```python
from build123d import *

# Parameters (mm, degrees)
BOSS_EXTRUDE1_DEPTH   = 10
SKETCH1_W             = 30
SKETCH1_H             = 3
BOSS_EXTRUDE1_2_DEPTH = 10
BOSS_EXTRUDE2_DEPTH   = 4.8
BOSS_EXTRUDE3_START   = 5.2
BOSS_EXTRUDE3_DEPTH   = 4.8
FILLET1_R             = 0.5
CUT_EXTRUDE1_REACH    = 55.298


with BuildPart() as part:
    # Sketch1 → Boss-Extrude1 (new, symmetric)
    with BuildSketch(Plane(origin=(0, 0, 0), x_dir=(0, 0, -1), z_dir=(1, 0, 0))):
        with BuildLine():
            Line((0, 13), (0, 11.2))
            Line((0, 11.2), (4.930378913, 10.768647738))
            Line((4.930378913, 10.768647738), (24, 13.896674439))
            Line((24, 13.896674439), (42, 13.896674439))
            ThreePointArc((42, 13.896674439), (43.5, 15.396674439), (42, 16.896674439))
            Line((42, 16.896674439), (23.755585281, 16.896674439))
            Line((23.755585281, 16.896674439), (0, 13))
        make_face()
    extrude(amount=BOSS_EXTRUDE1_DEPTH, both=True)



with BuildPart() as body_2:
    # Sketch1 → Boss-Extrude1 2 (new, symmetric)
    with BuildSketch(Plane(origin=(0, 0, 0), x_dir=(0, 0, -1), z_dir=(1, 0, 0))):
        with Locations((33, -2.5)):
            Rectangle(SKETCH1_W, SKETCH1_H)
    extrude(amount=BOSS_EXTRUDE1_2_DEPTH, both=True)


with BuildPart() as part_1:
    add(part.part)

    add(body_2.part)  # Boss-Extrude2 merges body 2
    # Sketch2 → Boss-Extrude2 (add, symmetric)
    with BuildSketch(Plane(origin=(0, 0, 0), x_dir=(0, 0, -1), z_dir=(1, 0, 0))):
        Polygon((30.537640136, 13.896674439), (45.434314575, -1), (46.565685425, -1), (31.669010986, 13.896674439), align=None)
    extrude(amount=BOSS_EXTRUDE2_DEPTH, both=True)

    # Sketch3 → Boss-Extrude3 (add)
    with BuildSketch(Plane(origin=(0, 0, 0), x_dir=(0, 0, -1), z_dir=(1, 0, 0)).offset(BOSS_EXTRUDE3_START)):
        Polygon((19.434314575, -1), (20.565685425, -1), (35.462359864, 13.896674439), (34.330989014, 13.896674439), align=None)
    boss_extrude3 = extrude(amount=BOSS_EXTRUDE3_DEPTH)

    # Mirror1: Boss-Extrude3 across plane
    add(boss_extrude3.mirror(Plane(origin=(0, 0, 0), x_dir=(0, 0, 1), z_dir=(1, 0, 0))))

    # Fillet1
    fillet1_edges = [part_1.edges().sort_by_distance(p)[0] for p in [
        (0, 13.896674439, -31.669010986),
        (0, 13.896674439, -30.537640136),
        (0, -1, -45.434314575),
        (0, -1, -46.565685425),
        (7.6, -1, -20.565685425),
        (7.6, 13.896674439, -35.462359864),
        (7.6, 13.896674439, -34.330989014),
        (7.6, -1, -19.434314575),
        (-7.6, -1, -20.565685425),
        (-7.6, -1, -19.434314575),
    ]]
    fillet(fillet1_edges, radius=FILLET1_R)

    # Sketch4 → Cut-Extrude1 (cut, up to next)
    with BuildSketch(Plane(origin=(0, 16.896674439, 0), x_dir=(1, 0, 0), z_dir=(0, 1, 0)), mode=Mode.PRIVATE) as cut_extrude1_sk1:
        Polygon((-3, 0), (-10, 26.585294569), (-10, 0), align=None)
    cut_extrude1_tool1 = extrude(cut_extrude1_sk1.sketch, amount=-CUT_EXTRUDE1_REACH, mode=Mode.PRIVATE) & part_1.part
    # Sketch4 → Cut-Extrude1 (cut, up to next)
    with BuildSketch(Plane(origin=(0, 16.896674439, 0), x_dir=(1, 0, 0), z_dir=(0, 1, 0)), mode=Mode.PRIVATE) as cut_extrude1_sk2:
        Polygon((3, 0), (10, 0), (10, 26.585294569), align=None)
    cut_extrude1_tool2 = extrude(cut_extrude1_sk2.sketch, amount=-CUT_EXTRUDE1_REACH, mode=Mode.PRIVATE) & part_1.part
    add(cut_extrude1_tool1.solids().sort_by_distance((-7.666667, 16.896674, -8.861765))[0], mode=Mode.SUBTRACT)
    add(cut_extrude1_tool2.solids().sort_by_distance((7.666667, 16.896674, -8.861765))[0], mode=Mode.SUBTRACT)


solid = part_1.part
```
Could you check a few things on this model? Use its own coordinates, in mm. A direction names the side the tool comes from. Coordinates: 2 decimals unless noted, no trailing zeros. Write each loop counter-clockwise with the first axis right and the second up, starting at its lowest first coordinate (ties: lowest second). Pieces come first, ordered by that corner, then holes. Notation, with made-up numbers: (57, -37.5) -> (116, -37.5) arc R32 ccw to (116, -11.5) -> close; hole circle Ø7 at (44.5, -20.75). An arc over 180 degrees is marked (long way). One line per question, with ' | ' between items. Start each with the question number.
1. Thinking about a two-plate mould opening in X: for faces 4 (the face through (-10, 7, -28)), 5 (the face through (5.2, 6, -27)), 6 (the face through (0.067, -0.699, -44.686)), 7 (the face through (-5.2, 6, -27)), which applies, pulls with the +X half, pulls with the -X half, needs draft (parallel to the pull), parting line crosses it, or undercut?
2. Please list where these lines run through material, in increasing order: line 1 along Y through (x, z) = (8, -29); line 2 along Y through (x, z) = (5.25, -37); line 3 along Y through (x, z) = (6, -31).
3. For faces 1 (the face through (6.55, 13.88, -13.48)), 2 (the face through (0.13, 12.66, -16.45)), 3 (the face through (-0.07, 13.58, -32.41)), which set-ups out of +Z, -Z, +X, -X, +Y, -Y let a thin tool reach every point of the face, with its end or its side?
4. If we section it at A-A (y = 9): Please give me the cut outline in (x, z).
5. If we section it at D-D (y = -1.5): Please give me the cut outline in (x, z).
6. Will these pins go through, and if not, where does the flat tip stop? P1, Ø8, axis at y = 0.5, z = -28, coming from the +X side; P2, Ø7.5, axis at y = 6.5, z = -40.5, coming from the +X side; P3, Ø8, axis at x = 2.5, y = 4.5, coming from the -Z side; P4, Ø1, axis at x = 5.5, y = 11.5, coming from the -Z side.
7. If we section it at C-C (z = -10): Please give me the cut outline in (x, y).
8. If we section it at B-B (x = -2.5): Please give me the cut outline in (y, z), and give its area (3 significant figures).
Return value:
1) face 4: pulls with the -X half | face 5: undercut | face 6: needs draft | face 7: undercut
2) line 1: y = -4 to -1, 7.43 to 8.57, 13.9 to 16.9 | line 2: y = -4 to -1, 13.9 to 16.9 | line 3: y = -4 to -1, 9.43 to 10.57, 13.9 to 16.9
3) face 1: +Z, +X, +Y | face 2: +X, -X | face 3: -Z, +X, -X
4) outline: (-10, -30.57) -> (-5.2, -30.57) -> (-5.2, -29.43) -> (-10, -29.43) -> close; (-4.8, -36.57) -> (4.8, -36.57) -> (4.8, -35.43) -> (-4.8, -35.43) -> close; (5.2, -30.57) -> (10, -30.57) -> (10, -29.43) -> (5.2, -29.43) -> close
5) outline: (-10, -48) -> (10, -48) -> (10, -18) -> (-10, -18) -> close
6) P1: stops at x = 10 | P2: stops at x = 4.8 | P3: stops at z = -45.07 | P4: stops at z = -33.57
7) outline: (-5.63, 11.6) -> (5.63, 11.6) -> (5.63, 14.64) -> (-5.63, 14.64) -> close
8) outline: (-4, -48) -> (-1, -48) -> (-1, -46.77) arc R0.5 cw to (-0.85, -46.42) -> (13.04, -32.52) arc R0.5 cw to (13.9, -32.88) -> (13.9, -42) arc R1.5 ccw to (16.9, -42) -> (16.9, -23.76) -> (13, 0) -> (11.2, 0) -> (10.77, -4.93) -> (13.9, -24) -> (13.9, -30.33) arc R0.5 cw to (13.75, -30.68) -> (-0.15, -44.58) arc R0.5 cw to (-1, -44.23) -> (-1, -18) -> (-4, -18) -> close | area: 235 mm²
